The model under review builds one solid part; all positions refer to its coordinate system, in mm. Coordinates: 2 decimals unless noted, no trailing zeros. Loops run counter-clockwise (first coordinate to the right, second up) from the corner with the lowest first, then second, coordinate; pieces in that order, holes last. Notation, with made-up numbers: (-30.75, 26) - (26.25, 26) arc R28 ccw to (26.25, 55) - close; hole circle Ø3 at (-38, 0). An arc over 180 degrees is marked (long way). Answer in a Markdown table with one row per item. Add a question column.
(1) We need section D-D on z = -8.5. Write out the cut boundary in (x, y).
(2) For P1, Ø1.5, axis at y = 1.5, z = 9.5, coming from the +X side; P2, Ø0.9, axis at x = -56, y = 1.5, coming from the +Z side; P3, Ø0.9, axis at x = -57.5, y = 1, coming from the -Z side, all flat-tipped, find the tip position at first contact; note any pin that passes through.
(3) For line 1 along X through (y, z) = (1.3, 0); line 2 along X through (y, z) = (0.3, 11), list the stretches that pass through material, from the lowest coordinate up.
(4) We need section A-A on x = 25. Write out the cut boundary in (y, z).
(5) We need section B-B on z = 0. Write out the cut boundary in (x, y), plus the area to 3 significant figures.
from build123d import *

# Parameters (mm, degrees)
CROQUIS1_R              = 2
SALIENTE_EXTRUIR1_DEPTH = 3


with BuildPart() as part:
    # Croquis1 → Saliente-Extruir1 (new body)
    with BuildSketch(Plane(origin=(0, 0, 0), x_dir=(1, 0, 0), z_dir=(0, 1, 0))):
        Polygon((55, 14.9), (55, 5.1), (58.2, 5.1), (58.2, -5.1), (55, -5.1), (55, -14.9), (58.2, -14.9), (58.2, -25.1), (55, -25.1), (55, -40), (-55, -40), (-55, -25.1), (-58.2, -25.1), (-58.2, -14.9), (-55, -14.9), (-55, -5.1), (-58.2, -5.1), (-58.2, 5.1), (-55, 5.1), (-55, 14.9), (-58.2, 14.9), (-58.2, 25.1), (-55, 25.1), (-55, 40), (55, 40), (55, 25.1), (58.2, 25.1), (58.2, 14.9), align=None)
        with Locations(Location((25, 0, 0), (0, 0, 270))):
            Circle(CROQUIS1_R, mode=Mode.SUBTRACT)
    extrude(amount=SALIENTE_EXTRUIR1_DEPTH)


solid = part.part
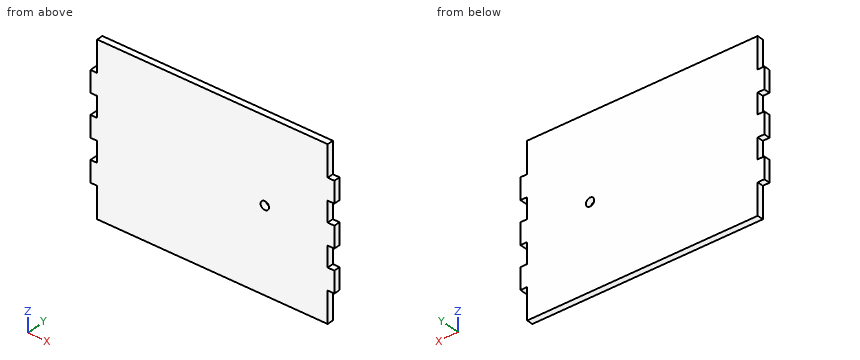
Outcome:
| question | item | result |
|---|---|---|
| 1 | outline | (-55, 0) - (55, 0) - (55, 3) - (-55, 3) - close |
| 2 | P1 | x = 55 |
| 2 | P2 | z = 25.1 |
| 2 | P3 | z = -25.1 |
| 3 | line 1 | -58.2 to 23, 27 to 58.2 |
| 3 | line 2 | -55 to 55 |
| 4 | outline | (0, -40) - (3, -40) - (3, -2) - (0, -2) - close; (0, 2) - (3, 2) - (3, 40) - (0, 40) - close |
| 5 | outline | (-58.2, 0) - (23, 0) - (23, 3) - (-58.2, 3) - close; (27, 0) - (58.2, 0) - (58.2, 3) - (27, 3) - close |
| 5 | area | 337 mm² |
